Design review of the part built by this model. Coordinates are the model's own, in mm. Face numbers are marked on the shaded views. A direction names the side the tool comes from. Give positions to 0.01 mm unless a question says otherwise; leave off trailing zeros. Order: outer loops, then holes, each group sorted by start corner. A loop starts at its lowest first (then second) coordinate and runs counter-clockwise, first axis right, second up.
```python
from build123d import *

# Parameters (mm, degrees)
SM_BASE_FLANGE_1_DEPTH = 465
SKETCH_4_W             = 54
SKETCH_4_H             = 180
CUT_EXTRUDE_2_DEPTH    = 710.542105868
HOLE_WIZARD_M21_D      = 2.4
HOLE_WIZARD_M21_DEPTH  = 5
HOLE_WIZARD_M21_TIP    = 0.721032743
HOLE_WIZARD_M22_D      = 2.4


# Sheet-metal steps are written as plain solids
with BuildPart() as part:
    # Sketch 1 → Базовая кромка1 (new body)
    with BuildSketch(Plane.XY):
        with BuildLine():
            Line((0, 0), (0, 273.5))
            ThreePointArc((0, 273.5), (0.146446609, 273.853553391), (0.5, 274))
            Line((0.5, 274), (457.5, 274))
            ThreePointArc((457.5, 274), (457.853553391, 273.853553391), (458, 273.5))
            Line((458, 273.5), (458, 0))
            Line((458, 0), (459, 0))
            Line((459, 0), (459, 273.5))
            ThreePointArc((459, 273.5), (458.560660172, 274.560660172), (457.5, 275))
            Line((457.5, 275), (0.5, 275))
            ThreePointArc((0.5, 275), (-0.560660172, 274.560660172), (-1, 273.5))
            Line((-1, 273.5), (-1, 0))
            Line((-1, 0), (0, 0))
        make_face()
    extrude(amount=SM_BASE_FLANGE_1_DEPTH)

    # Эскиз4 → Вырез-Вытянуть2 (cut, through all)
    with BuildSketch(Plane.ZY.offset(1)):
        with Locations((438, 185)):
            Rectangle(SKETCH_4_W, SKETCH_4_H)
    extrude(amount=-CUT_EXTRUDE_2_DEPTH, mode=Mode.SUBTRACT)

    # Отверстие с зазором M21
    with Locations(Plane(origin=(0, 275, 0), x_dir=(-1, 0, 0), z_dir=(0, 1, 0))):
        with Locations((-9, 403.5), (-31, 403.5), (-53, 403.5), (-75, 403.5), (-97, 403.5), (-119, 403.5), (-141, 403.5), (-163, 403.5), (-185, 403.5), (-207, 403.5), (-229, 403.5), (-251, 403.5), (-273, 403.5), (-295, 403.5), (-317, 403.5), (-339, 403.5), (-361, 403.5), (-383, 403.5), (-405, 403.5), (-427, 403.5), (-449, 403.5)):
            Hole(HOLE_WIZARD_M21_D / 2, depth=HOLE_WIZARD_M21_DEPTH)
            with Locations((0, 0, -(HOLE_WIZARD_M21_DEPTH + HOLE_WIZARD_M21_TIP / 2))):  # 118° drill point
                Cone(0, HOLE_WIZARD_M21_D / 2, HOLE_WIZARD_M21_TIP, mode=Mode.SUBTRACT)

    # Отверстие с зазором M22 (through all)
    with Locations(Plane(origin=(459, 0, 0), x_dir=(0, 0, -1), z_dir=(1, 0, 0))):
        with Locations((-403.5, 265), (-403.5, 245), (-403.5, 225), (-403.5, 205), (-403.5, 185), (-403.5, 165), (-403.5, 145), (-403.5, 125), (-403.5, 105), (-421, 87.5), (-441, 87.5)):
            Hole(HOLE_WIZARD_M22_D / 2)


solid = part.part
```
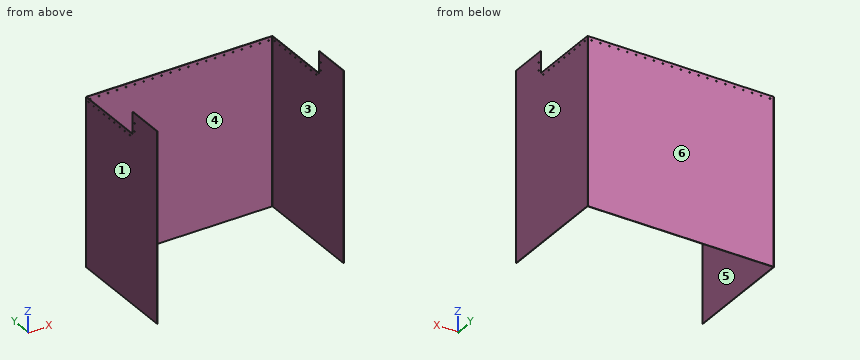
1. Take a section at C-C (y = 63). State the section outline as (x, z) points, then the cut area to 3 significant figures.
Recorded:
outline: (-1, 0) - (0, 0) - (0, 465) - (-1, 465) - close; (458, 0) - (459, 0) - (459, 465) - (458, 465) - close
area: 930 mm2
2. Take a section at D-D (x = 131.5). State the section outline as (y, z) points.
Recorded:
outline: (274, 0) - (275, 0) - (275, 411) - (274, 411) - close
3. For pin 1 (0.8 mm diameter, centred on x = -0.5, z = 435, fed in from +Y); pin 2 (3 mm diameter, centred on y = 225, z = 403.5, fed in from +X); pin 3 (3 mm diameter, centred on x = 75, z = 403.5, fed in from -Y), all flat-tipped, find the tip position at first contact; note any pin that passes through.
Recorded:
pin 1: stops at y = 95
pin 2: stops at x = 459
pin 3: stops at y = 274
4. Take a section at B-B (z = 155.5). State the section outline as (x, y) points.
Recorded:
outline: (-1, 0) - (0, 0) - (0, 273.5) arc R0.5 cw to (0.5, 274) - (457.5, 274) arc R0.5 cw to (458, 273.5) - (458, 0) - (459, 0) - (459, 273.5) arc R1.5 ccw to (457.5, 275) - (0.5, 275) arc R1.5 ccw to (-1, 273.5) - close
5. Machinability: for the marked faces 5 and 6, which of the approach directions +Z, -Z, +X, -X, +Y, -Y give a long, thin tool a straight path to every point of the face, cutting with its end or side? Answer none if there is none.
Recorded:
face 5: +Z, -Z, -Y
face 6: +Z, -Z, +X, -X, +Y
6. For line 1 along X through (y, z) = (137, 326); line 2 along Z through (x, y) = (458.7, 225); line 3 along Y through (x, z) = (412, 303), list the stretches that pass through material, from the lowest coordinate up.
Recorded:
line 1: x = -1 to 0, 458 to 459
line 2: z = 0 to 402.3, 404.7 to 411
line 3: y = 274 to 275
7. Draft analysis for pull direction X (two halves, no side actions). For the marked faces 1, 2, 3 and 4, state which applies: pulls with the +X half, pulls with the -X half, needs draft (parallel to the pull), parting line crosses it, or undercut.
Recorded:
face 1: pulls with the -X half
face 2: pulls with the +X half
face 3: undercut
face 4: undercut
8. Take a section at A-A (y = 198). State the section outline as (x, z) points.
Recorded:
outline: (-1, 0) - (0, 0) - (0, 411) - (-1, 411) - close; (458, 0) - (459, 0) - (459, 411) - (458, 411) - close
